Check sheet for the modelled part. Datum: model origin and axes. Units: mm. Round coordinates to 2 decimals unless told otherwise and drop trailing zeros. Loops run counter-clockwise (first coordinate to the right, second up) from the corner with the lowest first, then second, coordinate; pieces in that order, holes last. Notation, with made-up numbers: M 11.5,66 L 68.5,66 A27 ccw 68.5,91 Z; hole C 22,14.5 d4. An arc over 180 degrees is marked long. One line per question, with ' | ' between items. Start each with the question number.
(1) Section check B-B (y = 30). Record the boundary of the cut face in (x, z), and give its area (3 significant figures).
(2) Thickness scan on probe 1 along Z at (x, y) = (-1, 31); probe 2 along Y at (x, z) = (13.5, -11.5); probe 3 along Y at (x, z) = (-2.5, -5). Record the ranges inside material, lowest first. Write a range as [from, to].
(3) Go/stop test with flat-tipped pins: P1, Ø5, axis at x = -15.5, z = 1.5, coming from the -Y side; P2, Ø12, axis at x = 10, y = 1.5, coming from the +Z side; P3, Ø1.5, axis at x = -10, z = -14.5, coming from the +Y side. Record where each tip stops, or that it passes through.
(4) Section check C-C (x = 2). Record the boundary of the cut face in (y, z).
(5) Section check D-D (z = 9.5). Record the boundary of the cut face in (x, y), and give its area (3 significant figures).
(6) Section check A-A (z = 17). Record the boundary of the cut face in (x, y).
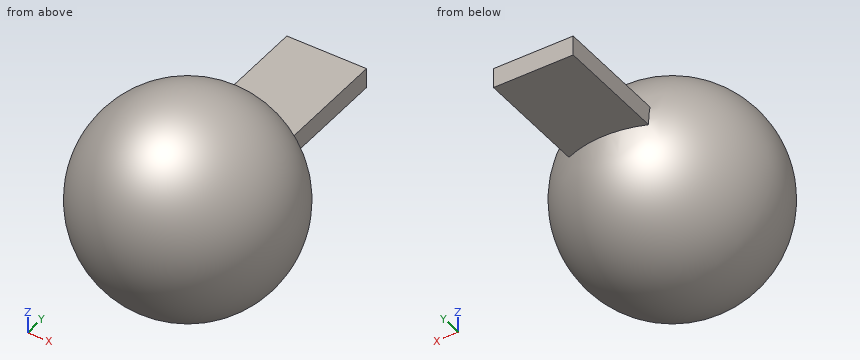
```python
from build123d import *

# Parameters (mm, degrees)
F3_DEPTH = 3.81
F4_W     = 15.193322
F4_H     = 3.81
F5_DEPTH = 50.8


with BuildPart() as f1:
    # F0 (on Front) → F1 (revolve)
    with BuildSketch(Plane.XZ):
        with BuildLine():
            ThreePointArc((-19.728339, 0), (0, -19.728339), (19.728339, 0))
            Line((19.728339, 0), (-19.728339, 0))
        make_face()
    revolve(axis=Axis((0, 0, 0), (-1, 0, 0)))

    # F2 (on Top) → F3 (join)
    with BuildSketch(Plane.XY):
        with BuildLine():
            Line((-7.596661, 39.821211), (-7.596661, 18.991655))
            ThreePointArc((-7.596661, 18.991655), (-0.00587, 19.47811), (7.596661, 19.236708))
            Line((7.596661, 19.236708), (7.596661, 39.821211))
            Line((7.596661, 39.821211), (-7.596661, 39.821211))
        make_face()
    extrude(amount=F3_DEPTH)

    # F4 (on face) → F5 (join)
    with BuildSketch(Plane(origin=(0, 39.821211, 0), x_dir=(-1, 0, 0), z_dir=(0, 1, 0))):
        with Locations((0, 1.905)):
            Rectangle(F4_W, F4_H)
    extrude(amount=-F5_DEPTH)


solid = f1.part
```
The answers:
1) outline: M -7.6,0 L 7.6,0 L 7.6,3.81 L -7.6,3.81 Z | area: 57.9 mm²
2) probe 1: [0, 3.81] | probe 2: [-8.64, 8.64] | probe 3: [-18.92, 18.92]
3) P1: y = -14.78 | P2: z = 19.3 | P3: y = 10.24
4) outline: M 19.25,3.81 A19.63 ccw long 19.63,0 L 39.82,0 L 39.82,3.81 Z
5) outline: C 0,0 d34.58 | area: 939 mm²
6) outline: C 0,0 d20.02
